Autodesk Inventor part; units mm, degrees
ref_plane "YZ Plane" through (0, 0, 0) normal (1, 0, 0) x (0, 1, 0)
ref_plane "XZ Plane" through (0, 0, 0) normal (0, 1, 0) x (-1, 0, 0)
ref_plane "XY Plane" through (0, 0, 0) normal (0, 0, 1) x (1, 0, 0)
sketch "Sketch1" plane through (0, 0, 0) normal (0, 0, 1) x (1, 0, 0)
  line L0 (0, 0) -> (76.2, 0)
  line L1 (76.2, 0) -> (76.2, -88.9)
  line L2 (76.2, -88.9) -> (50.8, -88.9)
  line L3 (50.8, -88.9) -> (50.8, -25.4)
  line L4 (50.8, -25.4) -> (0, -25.4)
  line L5 (0, -25.4) -> (0, 0)
  circle A0 centre (12.7, -12.7) radius 2.0701
  circle A1 centre (63.5, -30.1625) radius 2.0701
  circle A2 centre (63.5, -42.8625) radius 2.0701
  circle A3 centre (63.5, -55.5625) radius 2.0701
  circle A4 centre (63.5, -68.2625) radius 2.0701
  circle A5 centre (63.5, -80.9625) radius 2.0701
  circle A6 centre (25.4, -12.7) radius 2.0701
  circle A7 centre (38.1, -12.7) radius 2.0701
  circle A8 centre (50.8, -12.7) radius 2.0701
  circle A9 centre (63.5, -12.7) radius 2.0701
  dimension "d0" = 76.2
  dimension "d3" = 25.4
  dimension "d4" = 88.9
  dimension "d5" = 4.1402
  dimension "d6" = 12.7
  dimension "d7" = 12.7
  dimension "d18" = 12.7
  dimension "d23" = 12.7
  dimension "d27" = 4.7625
  dimension "d28" = 25.4
  dimension "d31" = 12.7
extrude "Extrusion1" add sketch "Sketch1" along normal blind 3.175
fillet "Fillet1" radius 3.175 6 edges at (0, 0, 1.5875) (0, -25.4, 1.5875) (50.8, -25.4, 1.5875) (50.8, -88.9, 1.5875) (76.2, -88.9, 1.5875) (76.2, 0, 1.5875)
properties part number "Roller Crossbar Gusset (Custom)" material "Aluminum 6061"
Can you work these out from the model? Positions are in its coordinate system, mm. A direction names the side the tool comes from. Coordinates: 2 decimals unless noted, no trailing zeros. Write each loop counter-clockwise with the first axis right and the second up, starting at its lowest first coordinate (ties: lowest second). Pieces come first, ordered by that corner, then holes.
Q1. If we mould it in two halves opening along X, with no side actions, what happens to faces 3 (the face through (64.46, -66.43, 1.57)), 4 (the face through (50.8, -58, 2)), 5 (the face through (76.2, -44, 2))? For each: +X half, -X half, draft (parallel to the pull), parting line (faces both ways), or undercut.
Results found:
face 3: undercut
face 4: -X half
face 5: +X half
Q2. Please list where these lines run through material, in increasing order: L1, parallel to Y at x = 25.4, z = 1.3; L2, parallel to Y at x = 47, z = 0.35; L3, parallel to X at y = -44.5, z = 0.85.
Results found:
L1: y = -25.4 to -14.77, -10.63 to 0
L2: y = -25.4 to 0
L3: x = 50.8 to 62.23, 64.77 to 76.2
Q3. Imagine slicing it at A-A, the plane x = 12. List the corners of the cut face in (y, z) for me (3 decimals).
Results found:
outline: (-25.4, 0) - (-14.648, 0) - (-14.648, 3.175) - (-25.4, 3.175) - close; (-10.752, 0) - (0, 0) - (0, 3.175) - (-10.752, 3.175) - close
Q4. Imagine slicing it at B-B, the plane y = -12.7. List the corners of the cut face in (x, z) for me (3 decimals), plus the area to 3 significant figures.
Results found:
outline: (0, 0) - (10.63, 0) - (10.63, 3.175) - (0, 3.175) - close; (14.77, 0) - (23.33, 0) - (23.33, 3.175) - (14.77, 3.175) - close; (27.47, 0) - (36.03, 0) - (36.03, 3.175) - (27.47, 3.175) - close; (40.17, 0) - (48.73, 0) - (48.73, 3.175) - (40.17, 3.175) - close; (52.87, 0) - (61.43, 0) - (61.43, 3.175) - (52.87, 3.175) - close; (65.57, 0) - (76.2, 0) - (76.2, 3.175) - (65.57, 3.175) - close
area: 176 mm2
Q5. Imagine slicing it at D-D, the plane x = 25.4. List the corners of the cut face in (y, z) for me (3 decimals).
Results found:
outline: (-25.4, 0) - (-14.77, 0) - (-14.77, 3.175) - (-25.4, 3.175) - close; (-10.63, 0) - (0, 0) - (0, 3.175) - (-10.63, 3.175) - close
Q6. Which directions (+Z, -Z, +X, -X, +Y, -Y) give clear straight access to the entire face, cutting with the end or side of a thin tool? Please do faces 1 (the face through (26.513, -14.446, 1.565)), 2 (the face through (26, -25.4, 2)).
Results found:
face 1: +Z, -Z
face 2: +Z, -Z, -X, -Y
Q7. For P1, Ø1.6, axis at y = -67, z = 1.5, coming from the -X side, with a flat end and sliding along its axis, tell me the tip position at first contact or that it passes through.
Results found:
P1: stops at x = 50.8
Q8. Imagine slicing it at C-C, the plane z = 2.05. Count the separate pieces of the cut face and the enclosed holes in it, plus the area to 3 significant figures.
Results found:
separate pieces: 1
enclosed holes: 10
area: 3,410 mm2
